Read the model definition and answer for the solid it produces. Units are mm, in the model's axes. Face numbers are marked on the shaded views. A direction names the side the tool comes from. Give positions to 0.01 mm unless a question says otherwise; leave off trailing zeros. Order: outer loops, then holes, each group sorted by start corner. A loop starts at its lowest first (then second) coordinate and runs counter-clockwise, first axis right, second up. Notation, with made-up numbers: (18.5, 4) - (65.5, 4) arc R20 ccw to (65.5, 20) - close; hole circle Ø7 at (84.5, -38). An arc over 180 degrees is marked (long way). Return JSON: item names as keys, results as strings.
```python
from build123d import *

# Parameters (mm, degrees)
EXTRUDE1_START     = -3.65
SKETCH1_R          = 3.5
EXTRUDE1_DEPTH     = 10
EXTRUDE2_START     = -6.35
SKETCH6_R          = 6
EXTRUDE2_DEPTH     = 2.7
CUT_EXTRUDE1_DEPTH = 2.025
CHAMFER1_SIZE      = 0.3375
CHAMFER2_SIZE      = 0.75


with BuildPart() as part:
    # Sketch1 → Extrude1 (new body)
    with BuildSketch(Plane.XY.offset(EXTRUDE1_START)):
        Circle(SKETCH1_R)
    extrude(amount=EXTRUDE1_DEPTH)

    # Sketch6 → Extrude2 (add)
    with BuildSketch(Plane.XY.offset(EXTRUDE2_START)):
        with Locations(Location((0, 0, 0), (0, 0, 180))):
            Circle(SKETCH6_R)
    extrude(amount=EXTRUDE2_DEPTH)

    # Sketch7 → Cut-Extrude1 (cut)
    with BuildSketch(Plane.XY.offset(-6.35)):
        Polygon((0, 2.598076211), (-2.25, 1.299038106), (-2.25, -1.299038106), (0, -2.598076211), (2.25, -1.299038106), (2.25, 1.299038106), align=None)
    extrude(amount=CUT_EXTRUDE1_DEPTH, mode=Mode.SUBTRACT)

    # Chamfer1
    chamfer1_edges = [part.edges().sort_by_distance(p)[0] for p in [
        (6, 0, -3.65),
        (6, 0, -6.35),
    ]]
    chamfer(chamfer1_edges, length=CHAMFER1_SIZE)

    # Chamfer2
    chamfer2_edges = [part.edges().sort_by_distance(p)[0] for p in [
        (-3.5, 0, 6.35),
    ]]
    chamfer(chamfer2_edges, length=CHAMFER2_SIZE)


solid = part.part
```
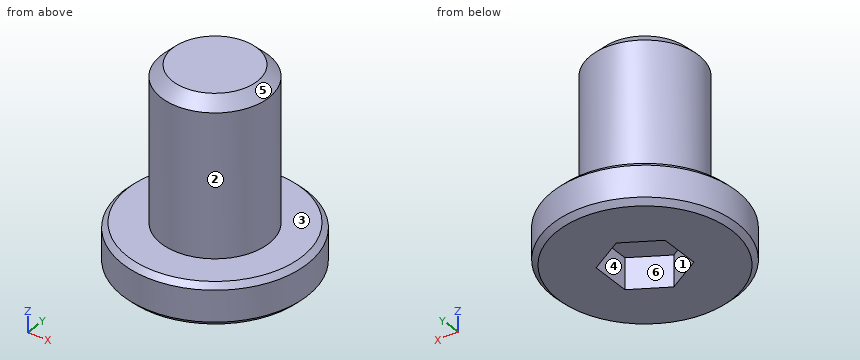
Q1. Given pin 1 (6 mm diameter, centred on x = 0, y = 1, fed in from -Z); pin 2 (1.5 mm diameter, centred on y = 1, z = -1, fed in from -X); pin 3 (6 mm diameter, centred on y = 4.5, z = 4.5, fed in from +X); pin 4 (0.6 mm diameter, centred on y = -0.5, z = -6, fed in from -X), each flat-ended and moving along its own axis, determine where each tip first touches the part or whether it passes through.
Values:
{"pin 1": "stops at z = -6.35", "pin 2": "stops at x = -3.49", "pin 3": "stops at x = 3.16", "pin 4": "stops at x = -6"}
Q2. For the marked faces 5 and 6, determine the directions among +Z, -Z, +X, -X, +Y, -Y from which every point of the face is accessible in a straight line to the end or side of a thin tool.
Values:
{"face 5": "+Z", "face 6": "-Z"}
Q3. A cutting plane is placed at A-A (z = -4.5). Write down the section's boundary in (x, y), and give its area (3 significant figures).
Values:
{"outline": "circle Ø12 at (0, 0); hole (-2.25, -1.3) - (0, -2.6) - (2.25, -1.3) - (2.25, 1.3) - (0, 2.6) - (-2.25, 1.3) - close", "area": "95.6 mm²"}
Q4. Consider L1, parallel to Z at x = -4, y = -2.25; L2, parallel to Y at x = -0.5, z = -5; L3, parallel to X at y = 1.75, z = -4.5. Determine where each line is inside the solid, lowest interval first.
Values:
{"L1": "z = -6.35 to -3.65", "L2": "y = -5.98 to -2.31, 2.31 to 5.98", "L3": "x = -5.74 to -1.47, 1.47 to 5.74"}
Q5. Determine the mould class of the marked faces 1, 2, 3 and 4 for opening direction X: released by +X, released by -X, zero draft, split by the parting line, or undercut.
Values:
{"face 1": "undercut", "face 2": "split by the parting line", "face 3": "zero draft", "face 4": "undercut"}
Q6. A cutting plane is placed at C-C (z = 1.5). Write down the section's boundary in (x, y).
Values:
{"outline": "circle Ø7 at (0, 0)"}
